The listing builds one solid part. Answer for the finished solid, in the listing's coordinates (mm). Face numbers are marked on the shaded views. Give positions to 0.01 mm unless a question says otherwise; leave off trailing zeros. Order: outer loops, then holes, each group sorted by start corner. A loop starts at its lowest first (then second) coordinate and runs counter-clockwise, first axis right, second up. Notation, with made-up numbers: (68.5, 54.5) - (78.5, 54.5) arc R27 cw to (78.5, 77.5) - close; hole circle Ø4 at (-6.5, -5). An arc over 180 degrees is marked (long way). Answer in a Markdown table with one row per item.
from build123d import *

# Parameters (mm, degrees)
ESQUISSE1_W             = 78
ESQUISSE1_H             = 13
BOSS_EXTRU_1_DEPTH      = 12
ESQUISSE2_W             = 78
ESQUISSE2_H             = 10.5
ENL_V_MAT_EXTRU_1_DEPTH = 11
D_GAGEMENT_M2_51_D      = 2.9
ESQUISSE5_W             = 31
ESQUISSE5_H             = 9
ENL_V_MAT_EXTRU_2_DEPTH = 41.908434338
D_GAGEMENT_M2_52_D      = 2.9
D_GAGEMENT_M2_52_DEPTH  = 24
D_GAGEMENT_M2_52_TIP    = 0.871247898
CONG_1_R                = 2


with BuildPart() as part:
    # Esquisse1 → Boss.-Extru.1 (new body)
    with BuildSketch(Plane.XY):
        Rectangle(ESQUISSE1_W, ESQUISSE1_H)
    extrude(amount=BOSS_EXTRU_1_DEPTH)

    # Esquisse2 → Enlèv. mat.-Extru.1 (cut)
    with BuildSketch(Plane(origin=(0, 6.5, 0), x_dir=(1, 0, 0), z_dir=(0, 1, 0))):
        with Locations((0, -5.25)):
            Rectangle(ESQUISSE2_W, ESQUISSE2_H)
    extrude(amount=-ENL_V_MAT_EXTRU_1_DEPTH, mode=Mode.SUBTRACT)

    # Dégagement M2.51 (through all)
    with Locations(Plane(origin=(0, -4.5, 0), x_dir=(1, 0, 0), z_dir=(0, 1, 0))):
        with Locations((33, -5.25), (-35, -5.25)):
            Hole(D_GAGEMENT_M2_51_D / 2)

    # Esquisse5 → Enlèv. mat.-Extru.2 (cut, through all)
    with BuildSketch(Plane(origin=(0, 0, 10.5), x_dir=(-1, 0, 0), z_dir=(0, 0, -1))):
        with Locations((-23.5, 2)):
            Rectangle(ESQUISSE5_W, ESQUISSE5_H)
    extrude(amount=-ENL_V_MAT_EXTRU_2_DEPTH, mode=Mode.SUBTRACT)

    # Dégagement M2.52
    with Locations(Plane.XY.offset(12)):
        with Locations((4, -2.7)):
            Hole(D_GAGEMENT_M2_52_D / 2, depth=D_GAGEMENT_M2_52_DEPTH)
            with Locations((0, 0, -(D_GAGEMENT_M2_52_DEPTH + D_GAGEMENT_M2_52_TIP / 2))):  # 118° drill point
                Cone(0, D_GAGEMENT_M2_52_D / 2, D_GAGEMENT_M2_52_TIP, mode=Mode.SUBTRACT)

    # Congé1
    cong_1_edges = [part.edges().sort_by_distance(p)[0] for p in [
        (39, -5.5, 0),
    ]]
    fillet(cong_1_edges, radius=CONG_1_R)


solid = part.part
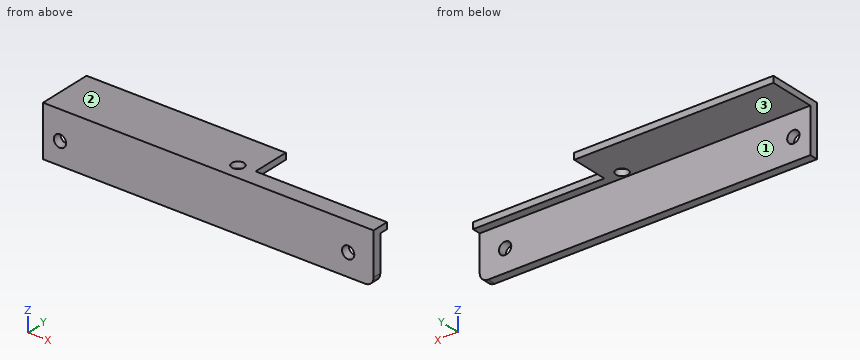
Item 1: Consider line 1 (X direction, y = -5.2, z = 5.25); line 2 (Z direction, x = -35, y = -5.2); line 3 (Y direction, x = -13.5, z = 1). Determine where each line is inside the solid, lowest interval first.
Answer block:
| item | result |
|---|---|
| line 1 | -39 to -36.45, -33.55 to 31.55, 34.45 to 39 |
| line 2 | 0 to 3.8, 6.7 to 12 |
| line 3 | -6.5 to -4.5 |
Item 2: Find section A-A on z = 5.25. Write down the section's boundary in (x, y), then the cut area to 3 significant figures.
Answer block:
| item | result |
|---|---|
| outline | (-39, -6.5) - (-36.45, -6.5) - (-36.45, -4.5) - (-39, -4.5) - close; (-33.55, -6.5) - (31.55, -6.5) - (31.55, -4.5) - (-33.55, -4.5) - close; (34.45, -6.5) - (39, -6.5) - (39, -4.5) - (34.45, -4.5) - close |
| area | 144 mm² |
Item 3: Each of these flat-tipped pins is pushed along its axis until it touches: P1, Ø3, axis at x = 8.5, z = 4, coming from the +Y side; P2, Ø2, axis at y = 0, z = 8, coming from the +X side; P3, Ø4, axis at x = 18.5, y = -1.5, coming from the -Z side. Where does it stop, or does it pass through?
Answer block:
| item | result |
|---|---|
| P1 | y = -4.5 |
| P2 | through |
| P3 | z = 10.5 |
Item 4: Find section B-B on x = -35. Write down the section's boundary in (y, z).
Answer block:
| item | result |
|---|---|
| outline | (-6.5, 0) - (-4.5, 0) - (-4.5, 3.8) - (-6.5, 3.8) - close; (-6.5, 6.7) - (-4.5, 6.7) - (-4.5, 10.5) - (6.5, 10.5) - (6.5, 12) - (-6.5, 12) - close |
Item 5: Determine the mould class of the marked faces 1, 2 and 3 for opening direction Z: pulls with the +Z half, pulls with the -Z half, needs draft (parallel to the pull), parting line crosses it, or undercut.
Answer block:
| item | result |
|---|---|
| face 1 | needs draft |
| face 2 | pulls with the +Z half |
| face 3 | pulls with the -Z half |
Item 6: Find section D-D on y = 4. Write down the section's boundary in (x, z).
Answer block:
| item | result |
|---|---|
| outline | (-39, 10.5) - (8, 10.5) - (8, 12) - (-39, 12) - close |
Item 7: Find section C-C on x = -1.5. Write down the section's boundary in (y, z), then the cut area to 3 significant figures.
Answer block:
| item | result |
|---|---|
| outline | (-6.5, 0) - (-4.5, 0) - (-4.5, 10.5) - (6.5, 10.5) - (6.5, 12) - (-6.5, 12) - close |
| area | 40.5 mm² |
